Geometry check sheet. Reference: the model listing, model coordinates, mm. Face numbers are marked on the shaded views. A direction names the side the tool comes from. Give positions to 0.01 mm unless a question says otherwise; leave off trailing zeros.
(1) Thickness scan on line 1 along X through (y, z) = (-60.5, 182.5); line 2 along Y through (x, z) = (-7, 181.5); line 3 along Z through (x, y) = (-11, -62). Record the ranges inside material, lowest first.
(2) Cross-section at A-A (x = -3). Count the separate pieces of the cut face and the enclosed holes in it, and give its area (3 significant figures).
(3) Mould release check, pull along Z, two halves, no side actions. Record for the marked faces 1 and 2: +Z half, -Z half, draft (parallel to the pull), parting line (faces both ways), or undercut.
(4) Depth check by flat-ended pin: P1, Ø12, axis at x = -14.5, z = 176.5, coming from the -Y side; P2, Ø2, axis at y = -61.5, z = 173, coming from the +X side; P3, Ø3, axis at y = -56.5, z = 177, coming from the +X side; P4, Ø2.5, axis at x = -13, z = 178.5, coming from the -Y side. Enter the tip coordinate at first touch or a pass-through.
(5) Tool access check on the marked faces 3 and 4. Record the directions out of +Z, -Z, +X, -X, +Y, -Y that give a thin tool (end or side, any length) a straight path to the whole face; none if there is none.
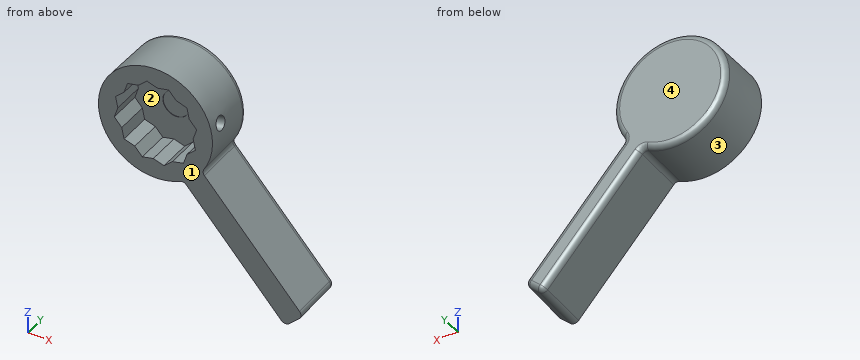
```python
from build123d import *

# Parameters (mm, degrees)
BOSS_EXTRU_1_DEPTH      = 10
BOSS_EXTRU_1_DRAFT      = 1
PER_AGE1_D              = 13
PER_AGE1_DEPTH          = 6
CONG_1_R                = 0.991556173
CONG_2_R                = 0.991556172
CONG_3_R                = 1
ENL_V_MAT_EXTRU_1_DEPTH = 6
ESQUISSE7_R             = 2.35630159
ENL_V_MAT_EXTRU_2_DEPTH = 0.1
TROU_TARAUD_M31_D       = 2.5
TROU_TARAUD_M31_DEPTH   = 8.5
TROU_TARAUD_M31_TIP     = 0.751075774


with BuildPart() as part:
    # Esquisse1 → Boss.-Extru.1 (with draft: the straight prism first)
    with BuildSketch(Plane(origin=(0, -53.604561249, 0), x_dir=(-1, 0, 0), z_dir=(0, 1, 0))):
        with BuildLine():
            Line((4.169645588, 172.151181972), (-13.92635809, 151.841438325))
            Line((-13.92635809, 151.841438325), (-10.939855184, 149.180460987))
            Line((-10.939855184, 149.180460987), (7.156148495, 169.490204634))
            ThreePointArc((7.156148495, 169.490204634), (18.83337708, 185.602358804), (4.169645588, 172.151181972))
        make_face()
    extrude(amount=-BOSS_EXTRU_1_DEPTH)
    # Boss.-Extru.1: the draft: its side faces are tilted about the plane it starts from
    boss_extru_1_sides = [part.faces().sort_by_distance(p)[0] for p in [
        (4.878356251, -58.604561249, 161.996310148),
        (12.433106637, -58.604561249, 150.510949656),
        (1.891853345, -58.604561249, 159.33533281),
        (-18.83337708, -58.604561249, 185.602358804),
    ]]
    draft(boss_extru_1_sides, Plane(origin=(0, -53.604561249, 0), x_dir=(-1, 0, 0), z_dir=(0, 1, 0)), BOSS_EXTRU_1_DRAFT)

    # Perçage1
    with Locations(Plane.XZ.offset(63.604561249)):
        with Locations((-12.180933736, 178.136101538)):
            Hole(PER_AGE1_D / 2, depth=PER_AGE1_DEPTH)

    # Congé1
    cong_1_edges = [part.edges().sort_by_distance(p)[0] for p in [
        (-7.174076316, -58.604557662, 169.379132828),
    ]]
    fillet(cong_1_edges, radius=CONG_1_R)

    # Congé2
    cong_2_edges = [part.edges().sort_by_distance(p)[0] for p in [
        (-4.057249498, -58.604557662, 172.156228913),
    ]]
    fillet(cong_2_edges, radius=CONG_2_R)

    # Congé3
    cong_3_edges = [part.edges().sort_by_distance(p)[0] for p in [
        (14.049579508, -58.604561249, 151.834335737),
        (12.433106637, -53.604561249, 150.510949656),
        (10.932752597, -58.604561249, 149.057239569),
        (5.137318128, -53.604561249, 161.705668665),
        (2.150815222, -53.604561249, 159.044691328),
        (-3.899737977, -53.604561249, 172.149959021),
        (-7.185946015, -53.604561249, 169.221944085),
        (-18.83337708, -53.604561249, 185.602358804),
    ]]
    fillet(cong_3_edges, radius=CONG_3_R)

    # Esquisse6 → Enlèv. mat.-Extru.1 (cut)
    with BuildSketch(Plane.XZ.offset(63.604561249)):
        Polygon((-6.577094401, 183.12912848), (-8.486502447, 183.760565155), (-9.824379984, 185.262109379), (-11.793694196, 184.854245557), (-13.703102242, 185.485682232), (-15.204646466, 184.147804695), (-17.173960678, 183.739940873), (-17.805397352, 181.830532827), (-19.306941577, 180.49265529), (-18.899077755, 178.523341078), (-19.530514429, 176.613933032), (-18.192636892, 175.112388808), (-17.78477307, 173.143074596), (-15.875365024, 172.511637922), (-14.537487487, 171.010093697), (-12.568173276, 171.417957519), (-10.658765229, 170.786520845), (-9.157221005, 172.124398382), (-7.187906794, 172.532262204), (-6.556470119, 174.44167025), (-5.054925895, 175.779547787), (-5.462789717, 177.748861998), (-4.831353042, 179.658270044), (-6.169230579, 181.159814269), align=None)
    extrude(amount=-ENL_V_MAT_EXTRU_1_DEPTH, mode=Mode.SUBTRACT)

    # Esquisse7 → Enlèv. mat.-Extru.2 (cut)
    with BuildSketch(Plane.XZ.offset(57.604561249)):
        with Locations(Location((-12.180933736, 178.136101538, 0), (0, 0, 270))):
            Circle(ESQUISSE7_R)
    extrude(amount=-ENL_V_MAT_EXTRU_2_DEPTH, mode=Mode.SUBTRACT)

    # Trou taraudé M31
    with Locations(Plane(origin=(30.587175126, -0.239784127, 3.6865788), x_dir=(-0.20280563003866656, 0, 0.9792190135126153), z_dir=(-0.9792190135126153, 0, -0.20280563003866656))):
        with Locations((179.497902827, -60.604561249)):
            Hole(TROU_TARAUD_M31_D / 2, depth=TROU_TARAUD_M31_DEPTH)
            with Locations((0, 0, -(TROU_TARAUD_M31_DEPTH + TROU_TARAUD_M31_TIP / 2))):  # 118° drill point
                Cone(0, TROU_TARAUD_M31_D / 2, TROU_TARAUD_M31_TIP, mode=Mode.SUBTRACT)


solid = part.part
```
Reply:
1. line 1: x = -21.31 to -17.58, -6.45 to -3.05
1. line 2: y = -57.6 to -53.6
1. line 3: z = 168.06 to 170.9, 185.02 to 188.21
2. separate pieces: 2
2. enclosed holes: 1
2. area: 139 mm2
3. face 1: draft
3. face 2: undercut
4. P1: stops at y = -63.6
4. P2: stops at x = -2.92
4. P3: stops at x = -2.11
4. P4: stops at y = -57.5
5. face 3: +Y
5. face 4: +Z, -Z, +X, -X, +Y
